Geometry: final body of the model. Coordinates: model frame, mm. Face numbers are marked on the shaded views. Coordinates: 2 decimals unless noted, no trailing zeros. Write each loop counter-clockwise with the first axis right and the second up, starting at its lowest first coordinate (ties: lowest second). Pieces come first, ordered by that corner, then holes. Notation, with made-up numbers: M 58,7.25 L 101,7.25 A33 cw 101,40.25 Z; hole C 82,64 d8. An arc over 180 degrees is marked long. Write item = value, one per line. Start each with the question number.
Item 1: Section C-C on y = -19.5. Output: boundary loops of the cut face in (x, z).
Item 2: Section B-B on z = 47.5. Output: boundary loops of the cut face in (x, y), plus the area to 3 significant figures.
Item 3: Section D-D on y = -67.5. Output: boundary loops of the cut face in (x, z).
Item 4: Ray query, L1, parallel to Y at x = 70, z = 17; L2, parallel to X at y = -55.5, z = 13.5; L3, parallel to X at y = -61.5, z = 28.5. Return the intervals inside material, ascending. Write a range as [from, to].
Item 5: Pull-direction query (X, two-part tool) for the marked faces 1, 2 and 3; classes: +X half, -X half, draft (parallel to the pull), parting line (faces both ways), or undercut.
Item 6: Section A-A on x = 64. Output: boundary loops of the cut face in (y, z).
Item 7: First-contact query: pin 1 Ø5 at (x, z) = (-16, 29.5) entering from +Y; pin 2 Ø18 at (x, y) = (-70, -60) entering from +Z; pin 3 Ø5.5 at (y, z) = (-78.5, 22) entering from -X; pin 4 Ø5.5 at (y, z) = (-78, 19) entering from +X. Flat tips, straight axial feed; report the tip coordinate or a pass-through.
from build123d import *

# Parameters (mm, degrees)
SKETCH2_R           = 10
BOSS_EXTRUDE1_DEPTH = 50


with BuildPart() as part:
    # Sketch2 → Boss-Extrude1 (new body)
    with BuildSketch(Plane.XY):
        with BuildLine():
            Line((-60, 0), (-90, 0))
            Line((-90, 0), (-90, -7.723724189))
            Line((-90, -7.723724189), (-90, -60))
            ThreePointArc((-90, -60), (-84.142135624, -74.142135624), (-70, -80))
            Line((-70, -80), (-60, -80))
            Line((-60, -80), (-60, -75))
            ThreePointArc((-60, -75), (-58.535533906, -71.464466094), (-55, -70))
            Line((-55, -70), (55, -70))
            ThreePointArc((55, -70), (58.535533906, -71.464466094), (60, -75))
            Line((60, -75), (60, -80))
            Line((60, -80), (70, -80))
            ThreePointArc((70, -80), (84.142135624, -74.142135624), (90, -60))
            Line((90, -60), (90, -7.723724189))
            Line((90, -7.723724189), (90, 0))
            Line((90, 0), (60, 0))
            ThreePointArc((60, 0), (0, -60), (-60, 0))
        make_face()
        with Locations((-70, -60)):
            Circle(SKETCH2_R, mode=Mode.SUBTRACT)
        with Locations(Location((70, -60, 0), (0, 0, 180))):
            Circle(SKETCH2_R, mode=Mode.SUBTRACT)
    extrude(amount=BOSS_EXTRUDE1_DEPTH)


solid = part.part
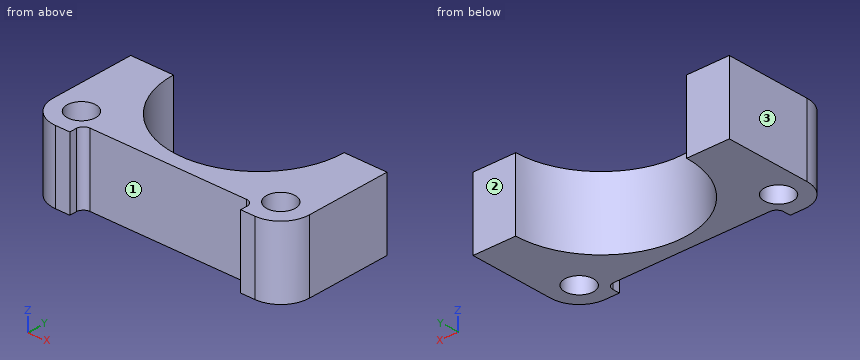
Responses:
q1.outline = M -90,0 L -56.74,0 L -56.74,50 L -90,50 Z; M 56.74,0 L 90,0 L 90,50 L 56.74,50 Z
q2.outline = M -90,-60 A20 ccw -70,-80 L -60,-80 L -60,-75 A5 cw -55,-70 L 55,-70 A5 cw 60,-75 L 60,-80 L 70,-80 A20 ccw 90,-60 L 90,0 L 60,0 A60 cw -60,0 L -90,0 Z; hole C -70,-60 d20; hole C 70,-60 d20
q2.area = 6,760 mm²
q3.outline = M -88.54,0 L -76.61,0 L -76.61,50 L -88.54,50 Z; M -63.39,0 L 63.39,0 L 63.39,50 L -63.39,50 Z; M 76.61,0 L 88.54,0 L 88.54,50 L 76.61,50 Z
q4.L1 = [-80, -70], [-50, 0]
q4.L2 = [-90, -78.93], [-61.07, -22.8], [22.8, 61.07], [78.93, 90]
q4.L3 = [-89.94, -79.89], [-60.11, 60.11], [79.89, 89.94]
q5.face_1 = undercut
q5.face_2 = draft
q5.face_3 = -X half
q6.outline = M -80,0 L -68,0 L -68,50 L -80,50 Z; M -52,0 L 0,0 L 0,50 L -52,50 Z
q7.pin_1 = -57.08
q7.pin_2 = through
q7.pin_3 = -82.33
q7.pin_4 = 82.94
